Verification items for the finished model (mm, model axes). Face numbers are marked on the shaded views. Round coordinates to 2 decimals unless told otherwise and drop trailing zeros. Order: outer loops, then holes, each group sorted by start corner. A loop starts at its lowest first (then second) coordinate and runs counter-clockwise, first axis right, second up. Notation, with made-up numbers: M 61,-4 L 70,-4 A33 cw 70,33 Z; hole C 47,48 d4. An arc over 180 degrees is marked long. Answer as a JSON object with one key per item and string values. Group by question number.
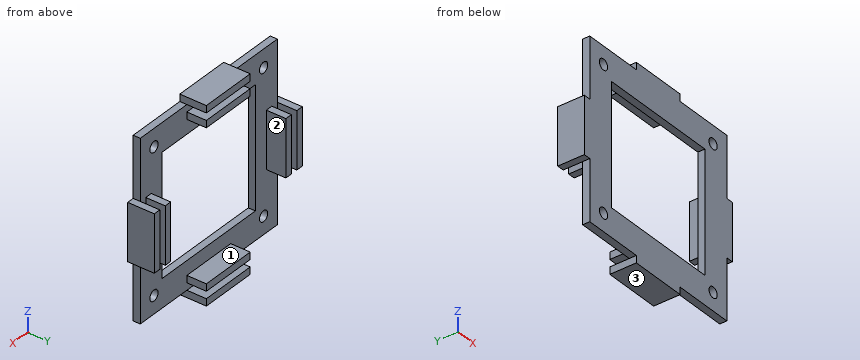
```python
from build123d import *

# Parameters (mm, degrees)
SKETCH1_W           = 50
SKETCH1_H           = 50
SKETCH1_W_2         = 34
SKETCH1_H_2         = 34
BOSS_EXTRUDE1_DEPTH = 2
SKETCH2_R           = 1.5
CUT_EXTRUDE1_DEPTH  = 2
SKETCH7_W           = 16
SKETCH7_H           = 2
SKETCH7_W_2         = 2
SKETCH7_H_2         = 16
BOSS_EXTRUDE4_DEPTH = 7.5


with BuildPart() as part:
    # Sketch1 → Boss-Extrude1 (new body)
    with BuildSketch(Plane(origin=(0, 0, 0), x_dir=(1, 0, 0), z_dir=(0, 1, 0))):
        Rectangle(SKETCH1_W, SKETCH1_H)
        Rectangle(SKETCH1_W_2, SKETCH1_H_2, mode=Mode.SUBTRACT)
    extrude(amount=BOSS_EXTRUDE1_DEPTH)

    # Sketch2 → Cut-Extrude1 (cut)
    with BuildSketch(Plane(origin=(0, 2, 0), x_dir=(1, 0, 0), z_dir=(0, 1, 0))):
        with Locations(Location((-20, 20, 0), (0, 0, 270))):
            Circle(SKETCH2_R)
        with Locations(Location((20, 20, 0), (0, 0, 270))):
            Circle(SKETCH2_R)
        with Locations(Location((20, -20, 0), (0, 0, 270))):
            Circle(SKETCH2_R)
        with Locations(Location((-20, -20, 0), (0, 0, 270))):
            Circle(SKETCH2_R)
    extrude(amount=-CUT_EXTRUDE1_DEPTH, mode=Mode.SUBTRACT)

    # Sketch7 → Boss-Extrude4 (add)
    with BuildSketch(Plane(origin=(0, 0, 0), x_dir=(1, 0, 0), z_dir=(0, 1, 0))):
        with Locations((0, 22)):
            Rectangle(SKETCH7_W, SKETCH7_H)
        with Locations((-26, 0)):
            Rectangle(SKETCH7_W_2, SKETCH7_H_2)
        with Locations((-22, 0)):
            Rectangle(SKETCH7_W_2, SKETCH7_H_2)
        with Locations((0, 26)):
            Rectangle(SKETCH7_W, SKETCH7_H)
        with Locations((22, 0)):
            Rectangle(SKETCH7_W_2, SKETCH7_H_2)
        with Locations((26, 0)):
            Rectangle(SKETCH7_W_2, SKETCH7_H_2)
        with Locations((0, -22)):
            Rectangle(SKETCH7_W, SKETCH7_H)
        with Locations((0, -26)):
            Rectangle(SKETCH7_W, SKETCH7_H)
    extrude(amount=BOSS_EXTRUDE4_DEPTH)


solid = part.part
```
Q1. Cross-section at D-D, the plane z = -20. Record the cut outline in (x, y).
Q2. Cross-section at A-A, the plane z = 12. Record the cut outline in (x, y), then the cut area to 3 significant figures.
Q3. Thickness scan on line 1 (X direction, y = 1.3, z = 20); line 2 (X direction, y = 3, z = 5.5). Record the ranges inside material, lowest first. Write a range as from..to.
Q4. Cross-section at C-C, the plane x = -20. Record the cut outline in (y, z).
Q5. Release check for a two-part mould opening along Z. For the marked faces 1, 2 and 3 record: released by +Z, released by -Z, zero draft, split by the parting line, or undercut.
Q6. Gauge pin test, flat ends, axial feed: pin 1 Ø1.6 at (y, z) = (1, -19.5) entering from -X; pin 2 Ø2 at (y, z) = (5.5, -21.5) entering from -X; pin 3 Ø0.6 at (y, z) = (4.5, 22) entering from +X. Record the tip position at first contact, or that the pin passes through.
Q7. Cross-section at B-B, the plane y = 4.25. Give the number of separate pieces and of enclosed holes in the cut face, then the cut area to 3 significant figures.
Conclusion:
{
 "1": {"outline": "M -25,0 L -21.5,0 L -21.5,2 L -25,2 Z; M -18.5,0 L 18.5,0 L 18.5,2 L -18.5,2 Z; M 21.5,0 L 25,0 L 25,2 L 21.5,2 Z"},
 "2": {"outline": "M -25,0 L -17,0 L -17,2 L -25,2 Z; M 17,0 L 25,0 L 25,2 L 17,2 Z", "area": "32.0 mm2"},
 "3": {"line 1": "-25..-21.5, -18.5..18.5, 21.5..25", "line 2": "-27..-25, -23..-21, 21..23, 25..27"},
 "4": {"outline": "M 0,-25 L 2,-25 L 2,-21.5 L 0,-21.5 Z; M 0,-18.5 L 2,-18.5 L 2,18.5 L 0,18.5 Z; M 0,21.5 L 2,21.5 L 2,25 L 0,25 Z"},
 "5": {"face 1": "undercut", "face 2": "zero draft", "face 3": "released by -Z"},
 "6": {"pin 1": "x = -25", "pin 2": "x = -8", "pin 3": "x = 8"},
 "7": {"separate pieces": "8", "enclosed holes": "0", "area": "256 mm2"}
}
